Autodesk Inventor part; units mm, degrees
ref_plane "YZ Plane" through (0, 0, 0) normal (1, 0, 0) x (0, 1, 0)
ref_plane "XZ Plane" through (0, 0, 0) normal (0, 1, 0) x (-1, 0, 0)
ref_plane "XY Plane" through (0, 0, 0) normal (0, 0, 1) x (1, 0, 0)
sketch "Sketch1" plane through (0, 0, 0) normal (0, 0, 1) x (1, 0, 0)
  line L0 (-240, 365) -> (240, 365)
  line L1 (240, 365) -> (240, -365)
  line L2 (240, -365) -> (-240, -365)
  line L3 (-240, -365) -> (-240, 365)
  line L4 (-225, 345) -> (225, 345)
  line L5 (225, 345) -> (225, -345)
  line L6 (225, -345) -> (-225, -345)
  line L7 (-225, -345) -> (-225, 345)
  point P0 (0, 0)
  dimension "d0" = 480
  dimension "d1" = 730
  dimension "d2" = 450
  dimension "d3" = 690
extrude "Extrusion1" add sketch "Sketch1" along normal blind 400
sketch "Sketch2" plane through (-240, 365, 0) normal (0, 1, 0) x (1, 0, 0)
  line L0 (20, 0) -> (20, -199)
  line L1 (20, 0) -> (219, 0) construction
  line L2 (20, -199) -> (460, -199)
  line L3 (460, -199) -> (460, 0)
  line L4 (15, 0) -> (465, 0)
  line L5 (465, -400) -> (15, -400)
  line L6 (20, -400) -> (20, -201)
  line L7 (15, 0) -> (15, -400)
  line L8 (20, -201) -> (460, -201)
  line L9 (20, -201) -> (460, -201) construction
  line L10 (460, -201) -> (460, -400)
  point P0 (240, 0)
extrude "Extrusion2" cut sketch "Sketch2" against normal blind 740 contours L4 L3 L2 L0
sketch "Sketch3" plane through (-240, 365, 400) normal (0, 1, 0) x (1, 0, 0)
  line L0 (20, 0) -> (20, 199)
  line L1 (20, 199) -> (460, 199)
  line L2 (460, 199) -> (460, 0)
  line L3 (15, 0) -> (465, 0)
  point P0 (240, 400)
  dimension "d15" = 199
  dimension "d16" = 440
extrude "Extrusion3" cut sketch "Sketch3" against normal blind 740
sketch "Sketch8" plane through (-225, -345, 0) normal (1, 0, 0) x (0, 0, -1)
  line L0 (-50, 527.5) -> (-70, 527.5)
  line L1 (-70, 527.5) -> (-70, 507.5)
  line L2 (-70, 507.5) -> (-50, 507.5)
  line L3 (-50, 507.5) -> (-50, 527.5)
  point P0 (0, 345)
  point P1 (0, 345)
extrude "Extrusion6" add sketch "Sketch8" along normal blind 460
sketch "Sketch9" plane through (-225, -345, 0) normal (1, 0, 0) x (0, 0, -1)
  line L0 (-50, 182.5) -> (-70, 182.5)
  line L1 (-70, 182.5) -> (-70, 162.5)
  line L2 (-70, 162.5) -> (-50, 162.5)
  line L3 (-50, 162.5) -> (-50, 182.5)
  point P0 (0, 345)
extrude "Extrusion7" add sketch "Sketch9" along normal blind 460
sketch "Sketch11" plane through (240, -365, 0) normal (1, 0, 0) x (0, 0, -1)
  line L0 (-400, 730) -> (-400, 0)
  line L1 (-400, 20) -> (-400, 710)
  line L2 (-400, 185.5) -> (-360, 185.5)
  line L3 (-360, 185.5) -> (-360, 125.5)
  line L4 (-360, 125.5) -> (-400, 125.5)
  line L5 (-400, 125.5) -> (-400, 185.5)
  point P0 (0, 365)
  point P1 (-400, 365)
extrude "Extrusion8" cut sketch "Sketch11" against normal blind 500
sketch "Sketch12" plane through (240, -365, 0) normal (1, 0, 0) x (0, 0, -1)
  line L0 (-400, 710) -> (-400, 185.5)
  line L1 (-400, 550.5) -> (-360, 550.5)
  line L2 (-360, 550.5) -> (-360, 490.5)
  line L3 (-360, 490.5) -> (-400, 490.5)
  line L4 (-400, 490.5) -> (-400, 550.5)
  point P0 (0, 365)
  point P1 (-400, 365)
extrude "Extrusion9" cut sketch "Sketch12" against normal blind 500
sketch "Sketch13" plane through (240, -365, 0) normal (1, 0, 0) x (0, 0, -1)
  line L0 (-360, 490.5) -> (-360, 550.5)
  point P0 (0, 365)
sketch "Sketch14" plane through (240, -365, 0) normal (1, 0, 0) x (0, 0, -1)
  point P0 (0, 365)
sketch "Sketch15" plane through (240, -365, 0) normal (1, 0, 0) x (0, 0, -1)
  point P0 (0, 365)
sketch "Sketch16" plane through (240, -365, 0) normal (1, 0, 0) x (0, 0, -1)
  point P0 (0, 365)
sketch "Sketch17" plane through (-225, -345, 0) normal (1, 0, 0) x (0, 0, -1)
  line L0 (-332.1423, 706.8149) -> (-312.1423, 706.8149)
  line L1 (-312.1423, 706.8149) -> (-312.1423, 686.8149)
  line L2 (-312.1423, 686.8149) -> (-332.1423, 686.8149)
  line L3 (-332.1423, 686.8149) -> (-332.1423, 706.8149)
  point P0 (0, 345)
  dimension "d43" = 20
  dimension "d44" = 20
extrude "Extrusion10" add sketch "Sketch17" along normal blind 450
sketch "Sketch18" plane through (-225, 162.5, 70) normal (0, 0, 1) x (1, 0, 0)
  line L0 (0, 20) -> (450, 20)
  line L1 (0, -345) -> (450, -345)
  line L2 (60, 20) -> (380, 20)
  line L3 (380, 20) -> (380, -345)
  line L4 (380, -345) -> (60, -345)
  line L5 (60, -345) -> (60, 20)
  point P0 (225, -162.5)
  dimension "d47" = 320
extrude "Extrusion11" add sketch "Sketch18" along normal blind 5
sketch "Sketch19" plane through (-225, 162.5, 75) normal (0, 0, 1) x (1, 0, 0)
  line L0 (175, -112.5) -> (275, -112.5)
  line L1 (275, -112.5) -> (275, -212.5)
  line L2 (275, -212.5) -> (175, -212.5)
  line L3 (175, -212.5) -> (175, -112.5)
  point P0 (225, -162.5)
  dimension "d50" = 100
  dimension "d51" = 100
extrude "Extrusion12" add sketch "Sketch19" along normal blind 5
sketch "Sketch20" plane through (-225, 162.5, 80) normal (0, 0, 1) x (1, 0, 0)
  circle A0 centre (200, -162.5) radius 5.5
  point P0 (225, -162.5)
  dimension "d54" = 11
sketch "Sketch21" plane through (-225, 162.5, 80) normal (0, 0, 1) x (1, 0, 0)
  circle A0 centre (250, -162.5) radius 5.5
  point P0 (225, -162.5)
  dimension "d57" = 11
properties part number "stand2.0"
Read the model definition and answer for the solid it produces. Units are mm, in the model's axes. A direction names the side the tool comes from. Coordinates: 2 decimals unless noted, no trailing zeros. Order: outer loops, then holes, each group sorted by start corner. A loop starts at its lowest first (then second) coordinate and runs counter-clockwise, first axis right, second up. Notation, with made-up numbers: M 19.5,-38.75 L 24.5,-38.75 A23 ccw 24.5,-14.75 Z; hole C 5,-5 d4. An arc over 180 degrees is marked long. Put each result on its own line as item: value. Start each with the question number.
Item 1: For faces 4 (the face through (233, -179.5, 380)), 5 (the face through (-3, -355, 199)), 6 (the face through (-7, 2, 70)), determine the directions among +Z, -Z, +X, -X, +Y, -Y from which every point of the face is accessible in a straight line to the end or side of a thin tool.
Item 2: Section A-A, the plane y = -110 is taken. Determine the outline of the cut face in (x, z), plus the area to 3 significant figures.
Item 3: Section D-D, the plane y = 258 is taken. Determine the outline of the cut face in (x, z).
Item 4: Consider probe 1 along X at (y, z) = (-163, 216.5); probe 2 along Z at (x, y) = (-79, 144); probe 3 along Z at (x, y) = (164.5, 168.5). Determine where each line is inside the solid, lowest interval first. Write a range as [from, to].
Item 5: Given pin 1 Ø10 at (x, y) = (-10.5, 355.5) entering from -Z; pin 2 Ø22 at (x, z) = (0.5, 55.5) entering from -Y; pin 3 Ø4 at (x, y) = (-41, -65.5) entering from +Z, each flat-ended and moving along its own axis, determine where each tip first touches the part or whether it passes through.
Item 6: Section B-B, the plane z = 247.5 is taken. Determine the outline of the cut face in (x, y).
Item 7: Section C-C, the plane x = 14.5 is taken. Determine the outline of the cut face in (y, z).
Item 8: The mould has two halves that part along Z. Classify faces 1 (the face through (190, -172, 70)), 2 (the face through (-232, 185.5, 380)), 3 (the face through (220, 355, 299)): +Z half, -Z half, draft (parallel to the pull), parting line (faces both ways), or undercut.
Computed:
1. face 4: +Z, +X, -X
1. face 5: -Z, +Y, -Y
1. face 6: -Z
2. outline: M -240,0 L -225,0 L -225,400 L -240,400 Z; M -165,70 L 155,70 L 155,75 L -165,75 Z; M 225,0 L 240,0 L 240,400 L 225,400 Z
2. area: 13,600 mm2
3. outline: M -240,0 L -225,0 L -225,400 L -240,400 Z; M 225,0 L 240,0 L 240,400 L 225,400 Z
4. probe 1: x = [-240, -225], [225, 240]
4. probe 2: z = [70, 75]
4. probe 3: z = [50, 70]
5. pin 1: stops at z = 199
5. pin 2: stops at y = -182.5
5. pin 3: stops at z = 75
6. outline: M -240,-365 L -220,-365 L -220,-345 L -225,-345 L -225,345 L -220,345 L -220,365 L -240,365 Z; M 220,-365 L 240,-365 L 240,365 L 220,365 L 220,345 L 225,345 L 225,-345 L 220,-345 Z
7. outline: M -365,199 L -345,199 L -345,201 L -365,201 Z; M -182.5,50 L -162.5,50 L -162.5,70 L 162.5,70 L 162.5,50 L 182.5,50 L 182.5,75 L 50,75 L 50,80 L -50,80 L -50,75 L -182.5,75 Z; M 341.81,312.14 L 361.81,312.14 L 361.81,332.14 L 341.81,332.14 Z; M 345,199 L 365,199 L 365,201 L 345,201 Z
8. face 1: +Z half
8. face 2: draft
8. face 3: undercut
